Geometry check sheet. Reference: drawing and pictorial views, mm from the part's lowest x, y, z. A direction names the side the tool comes from. Give positions to 0.01 mm unless a question says otherwise; leave off trailing zeros. Order: outer loops, then holes, each group sorted by start corner. A loop starts at its lowest first (then second) coordinate and runs counter-clockwise, first axis right, second up.
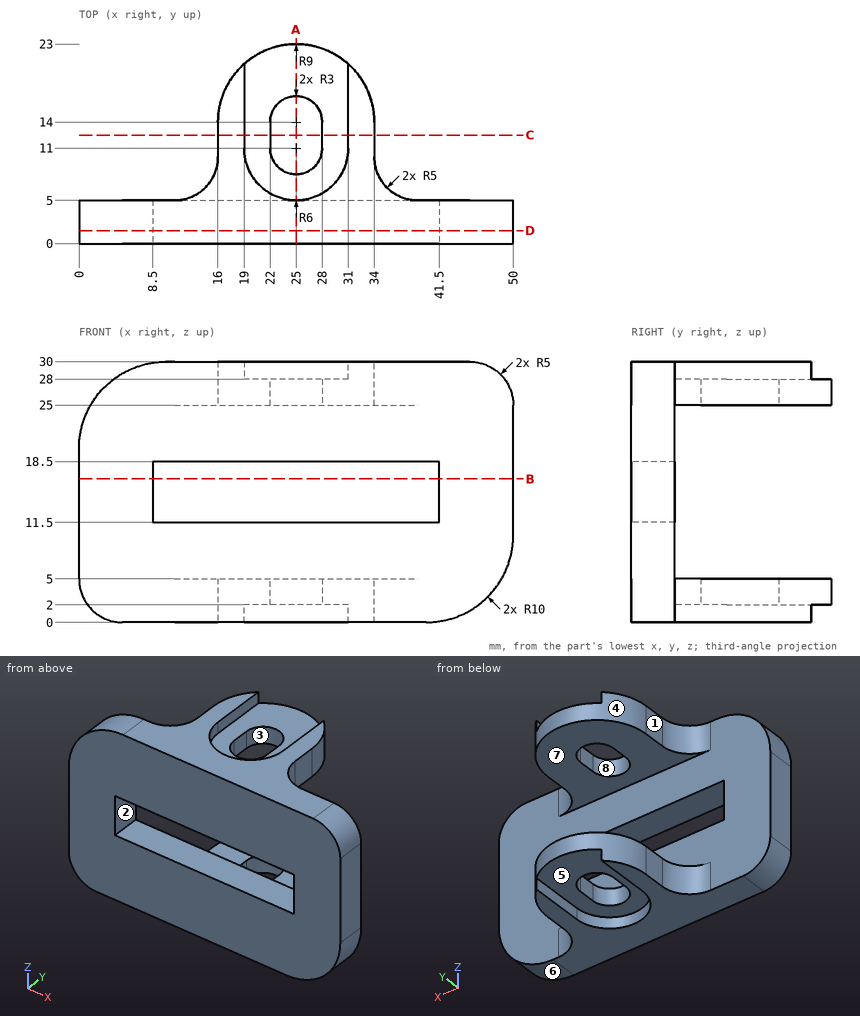
(1) Cross-section at B-B on z = 16.5. Enter the section's corners in (x, y).
Response values:
outline: (0, 0) - (8.5, 0) - (8.5, 5) - (0, 5) - close; (41.5, 0) - (50, 0) - (50, 5) - (41.5, 5) - close
(2) Material ranges on L1, parallel to Z at x = 26.5, y = 21.5; L2, parallel to X at y = 13.25, z = 28.5; L3, parallel to Z at x = 31, y = 3, recorded low to high.
Response values:
L1: z = 2 to 5, 25 to 28
L2: x = 16 to 19, 31 to 34
L3: z = 0 to 11.5, 18.5 to 30
(3) Cross-section at C-C on y = 12.5. Enter the section's corners in (x, z).
Response values:
outline: (16, 0) - (19, 0) - (19, 2) - (22, 2) - (22, 5) - (16, 5) - close; (16, 25) - (22, 25) - (22, 28) - (19, 28) - (19, 30) - (16, 30) - close; (28, 2) - (31, 2) - (31, 0) - (34, 0) - (34, 5) - (28, 5) - close; (28, 25) - (34, 25) - (34, 30) - (31, 30) - (31, 28) - (28, 28) - close
(4) Set-up check for the marked faces 1, 2, 3, 4 and 5: record each of +Z, -Z, +X, -X, +Y, -Y from which the full face is reachable in a straight line by a thin tool's end or side.
Response values:
face 1: +Z, -Z, -X, +Y
face 2: +Y, -Y
face 3: +Z, -Z
face 4: +Z, -Z, +Y
face 5: -Z, +Y
(5) Cross-section at A-A on x = 25. Enter the section's corners in (y, z), then the cut area to 3 significant figures.
Response values:
outline: (0, 0) - (5, 0) - (5, 2) - (8, 2) - (8, 5) - (5, 5) - (5, 11.5) - (0, 11.5) - close; (0, 18.5) - (5, 18.5) - (5, 25) - (8, 25) - (8, 28) - (5, 28) - (5, 30) - (0, 30) - close; (17, 2) - (23, 2) - (23, 5) - (17, 5) - close; (17, 25) - (23, 25) - (23, 28) - (17, 28) - close
area: 169 mm2
(6) Release check for a two-part mould opening along Z. For the marked faces 6, 7 and 8 record: released by +Z, released by -Z, zero draft, split by the parting line, or undercut.
Response values:
face 6: released by -Z
face 7: undercut
face 8: zero draft
(7) Cross-section at D-D on y = 1.5. Enter the section's corners in (x, z).
Response values:
outline: (0, 5) arc R5 ccw to (5, 0) - (40, 0) arc R10 ccw to (50, 10) - (50, 25) arc R5 ccw to (45, 30) - (10, 30) arc R10 ccw to (0, 20) - close; hole (8.5, 11.5) - (41.5, 11.5) - (41.5, 18.5) - (8.5, 18.5) - close
(8) Gauge pin test, flat ends, axial feed: pin 1 Ø3 at (x, y) = (40, 7.5) entering from -Z; pin 2 Ø3 at (y, z) = (12.5, 3.5) entering from -X; pin 3 Ø3 at (x, y) = (27.5, 19) entering from +Z; pin 4 Ø0.6 at (y, z) = (18, 1) entering from -X. Record the tip position at first contact, or that the pin passes through.
Response values:
pin 1: passes through
pin 2: stops at x = 16
pin 3: stops at z = 28
pin 4: stops at x = 16.8
